The listing builds one solid part. Answer for the finished solid, in the listing's coordinates (mm). Face numbers are marked on the shaded views. A direction names the side the tool comes from. Round coordinates to 2 decimals unless told otherwise and drop trailing zeros. Write each loop counter-clockwise with the first axis right and the second up, starting at its lowest first coordinate (ties: lowest second). Pieces come first, ordered by that corner, then holes.
Item 1: Find section A-A on z = 0. Give the vertices of the cut face in (x, y), then the cut area to 3 significant figures.
Item 2: For a pull along X with two mould halves and no side action, classify the marked faces 5, 6 and 7 as +X half, -X half, draft (parallel to the pull), parting line (faces both ways), or undercut.
Item 3: Find section B-B on x = 0. Give the vertices of the cut face in (y, z).
Item 4: A tool of negligible diameter and unlimited length cuts with its end or side. For the marked faces 1, 2, 3 and 4, from which of +Z, -Z, +X, -X, +Y, -Y can it reach the whole face along a straight path? Write none if from no direction.
Item 5: Each of these flat-tipped pins is pushed along its axis until it touches: pin 1 (10 mm diameter, centred on x = -9, y = -30, fed in from +Z); pin 2 (8 mm diameter, centred on y = -45, z = 5, fed in from -X); pin 3 (3 mm diameter, centred on x = 15, y = -33.5, fed in from -Z). Where does it stop, or does it pass through?
Item 6: Find the intervals of material crossed by probe 1 along X at (y, z) = (-23, 23); probe 2 along Z at (x, y) = (18.5, -21); probe 3 along Z at (x, y) = (-9.5, -5.5), in increasing order.
Item 7: Find section C-C on y = -40. Give the vertices of the cut face in (x, z).
```python
from build123d import *

# Parameters (mm, degrees)
F0_R     = 25.6
F1_DEPTH = 30
F3_DEPTH = 30
F4_COUNT = 18
F5_R     = 22.5
F6_DEPTH = 20
F8_DEPTH = 50.001
F9_R     = 0.2


with BuildPart() as f1:
    # F0 (on Front) → F1 (new body)
    with BuildSketch(Plane.XZ):
        Circle(F0_R)
    extrude(amount=F1_DEPTH)

    # F2 (on Front) → F3 (join, through all)
    with BuildSketch(Plane.XZ):
        with BuildLine():
            ThreePointArc((-2.5717175805, 25.4704980062), (0, 25.6), (2.5717175805, 25.4704980062))
            ThreePointArc((2.5717175805, 25.4704980062), (2.0656887709, 27.8468218747), (0.9139195769, 29.9860759521))
            ThreePointArc((0.9139195769, 29.9860759521), (0, 30), (-0.9139195769, 29.9860759521))
            ThreePointArc((-0.9139195769, 29.9860759521), (-2.0656887709, 27.8468218747), (-2.5717175805, 25.4704980062))
        make_face()
    extrude(amount=F3_DEPTH)

    # F4: F1 ×18 about axis
    f4_axis = Axis((0, 0, 0), (0, 1, 0))


with BuildPart() as f1_1:
    add(f1.part)
    for i in range(1, F4_COUNT):
        add(f1.part.rotate(f4_axis, i * 360 / F4_COUNT))

    # F5 (on face) → F6 (join)
    with BuildSketch(Plane.XZ.offset(30)):
        Circle(F5_R)
    extrude(amount=F6_DEPTH)

    # F7 (on Front) → F8 (cut, through all)
    with BuildSketch(Plane.XZ):
        with BuildLine():
            Line((4, 15.8), (-4, 15.8))
            Line((-4, 15.8), (-4, 11.8427192823))
            ThreePointArc((-4, 11.8427192823), (0, -12.5), (4, 11.8427192823))
            Line((4, 11.8427192823), (4, 15.8))
        make_face()
    extrude(amount=F8_DEPTH, mode=Mode.SUBTRACT)

    # F9
    f9_edges = [f1_1.edges().sort_by_distance(p)[0] for p in [
        (-4, -25, 15.8),
        (4, -25, 15.8),
    ]]
    fillet(f9_edges, radius=F9_R)


solid = f1_1.part
```
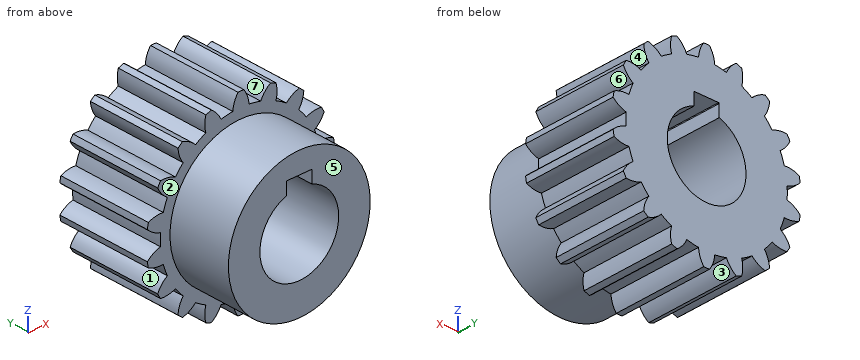
Check values:
1. outline: (-25.6, -30) - (-22.5, -30) - (-22.5, -50) - (-12.5, -50) - (-12.5, 0) - (-25.6, 0) - close; (12.5, -50) - (22.5, -50) - (22.5, -30) - (25.6, -30) - (25.6, 0) - (12.5, 0) - close
1. area: 1,190 mm2
2. face 5: draft
2. face 6: +X half
2. face 7: undercut
3. outline: (-50, -22.5) - (-30, -22.5) - (-30, -30) - (0, -30) - (0, -12.5) - (-50, -12.5) - close; (-50, 15.8) - (0, 15.8) - (0, 30) - (-30, 30) - (-30, 22.5) - (-50, 22.5) - close
4. face 1: -X, +Y, -Y
4. face 2: -Y
4. face 3: -Z, +Y, -Y
4. face 4: +X, +Y, -Y
5. pin 1: stops at z = 28.49
5. pin 2: stops at x = -22.48
5. pin 3: stops at z = -18
6. probe 1: x = -19.26 to -16.97, -11.24 to 11.24, 16.97 to 19.26
6. probe 2: z = -23.54 to -18.08, -17.69 to 17.69, 18.08 to 23.54
6. probe 3: z = -28.46 to -8.12, 8.12 to 28.46
7. outline: circle Ø45 at (0, 0); hole (-4, 11.84) arc R12.5 ccw (long way) to (4, 11.84) - (4, 15.6) arc R0.2 ccw to (3.8, 15.8) - (-3.8, 15.8) arc R0.2 ccw to (-4, 15.6) - close
